from build123d import *

# Parameters (mm, degrees)
F0_W     = 12.7
F0_H     = 25.4
F1_DEPTH = 76.2
F2_W     = 38.1
F2_H     = 12.7
F3_DEPTH = 50.801
F5_DEPTH = 50.801


with BuildPart() as f1:
    # F0 (on Right) → F1 (new body)
    with BuildSketch(Plane.YZ):
        Polygon((38.1, 38.1), (0, 0), (38.1, 0), (38.1, 25.4), align=None)
        with Locations((44.45, 12.7)):
            Rectangle(F0_W, F0_H)
        Polygon((38.1, 50.8), (38.1, 38.1), (38.1, 25.4), (50.8, 25.4), (50.8, 50.8), align=None)
    extrude(amount=F1_DEPTH)

    # F2 (on face) → F3 (cut, through all)
    with BuildSketch(Plane(origin=(0, 0, 0), x_dir=(1, 0, 0), z_dir=(0, 0, -1))):
        with Locations((38.1, -6.35)):
            Rectangle(F2_W, F2_H)
    extrude(amount=-F3_DEPTH, mode=Mode.SUBTRACT)

    # F4 (on face) → F5 (cut, through all)
    with BuildSketch(Plane(origin=(0, 50.8, 0), x_dir=(-1, 0, 0), z_dir=(0, 1, 0))):
        Polygon((-76.2, 38.1), (-63.5, 38.1), (-50.8, 50.8), (-76.2, 50.8), align=None)
        Polygon((-25.4, 50.8), (-12.7, 38.1), (0, 38.1), (0, 50.8), align=None)
        Polygon((0, 38.1), (-12.7, 38.1), (0, 25.4), align=None)
        Polygon((-76.2, 25.4), (-63.5, 38.1), (-76.2, 38.1), align=None)
    extrude(amount=-F5_DEPTH, mode=Mode.SUBTRACT)


solid = f1.part
Read the model definition and answer for the solid it produces. Units are mm, in the model's axes. A direction names the side the tool comes from. Round coordinates to 2 decimals unless told otherwise and drop trailing zeros. Write each loop counter-clockwise with the first axis right and the second up, starting at its lowest first coordinate (ties: lowest second). Pieces come first, ordered by that corner, then holes.
1. The part is cut by section A-A, the plane y = 35.5. Determine the outline of the cut face in (x, z).
2. Which of the six approach directions +Z, -Z, +X, -X, +Y, -Y give full straight-line access (tool end or side, diameter ignored) to faces 4 (the face through (38, 38.1, 43)), 5 (the face through (66.5, 41.1, 35.1)), 6 (the face through (19.05, 8, 5))?
3. Determine the mould class of faces 1 (the face through (38, 50.8, 19)), 2 (the face through (76.2, 31, 13)), 3 (the face through (38, 12.7, 6)) for opening direction X: pulls with the +X half, pulls with the -X half, needs draft (parallel to the pull), parting line crosses it, or undercut.
4. Given pin 1 Ø14 at (x, z) = (47.5, 45.5) entering from -Y; pin 2 Ø1.5 at (x, y) = (65, 14.5) entering from +Z; pin 3 Ø4 at (y, z) = (6.5, 7) entering from -X; pin 4 Ø6 at (x, y) = (18.5, 15.5) entering from +Z, each flat-ended and moving along its own axis, determine where each tip first touches the part or whether it passes through.
5. The part is cut by section D-D, the plane y = 47. Determine the outline of the cut face in (x, z), then the cut area to 3 significant figures.
6. The part is cut by section C-C, the plane z = 32. Determine the outline of the cut face in (x, y), then the cut area to 3 significant figures.
7. Straight lines are drawn through the part: L1, parallel to Y at x = 20.5, z = 39; L2, parallel to Y at x = 43, z = 8; L3, parallel to X at y = 38.5, z = 45. For each, find the intervals that lie inside material, in ascending order.
8. The part is cut by section B-B, the plane x = 14.5. Determine the outline of the cut face in (y, z), then the cut area to 3 significant figures.
Values:
1. outline: (0, 0) - (76.2, 0) - (76.2, 25.4) - (66.1, 35.5) - (10.1, 35.5) - (0, 25.4) - close
2. face 4: +Z, +X, -X, -Y
2. face 5: +Z, +X, +Y, -Y
2. face 6: +Z, -Z, -Y
3. face 1: needs draft
3. face 2: pulls with the +X half
3. face 3: undercut
4. pin 1: stops at y = 38.1
4. pin 2: stops at z = 15.25
4. pin 3: stops at x = 0
4. pin 4: stops at z = 18.5
5. outline: (0, 0) - (76.2, 0) - (76.2, 25.4) - (50.8, 50.8) - (25.4, 50.8) - (0, 25.4) - close
5. area: 3,230 mm2
6. outline: (6.6, 32) - (69.6, 32) - (69.6, 50.8) - (6.6, 50.8) - close
6. area: 1,180 mm2
7. L1: y = 38.1 to 50.8
7. L2: y = 12.7 to 50.8
7. L3: x = 19.6 to 56.6
8. outline: (0, 0) - (50.8, 0) - (50.8, 39.9) - (38.1, 39.9) - (38.1, 38.1) - close
8. area: 1,230 mm2
